Here's the drawing with two shaded views (mm, measured from the low corner). I have some questions. Round coordinates to 2 decimals unless told otherwise and drop trailing zeros. Order: outer loops, then holes, each group sorted by start corner. A loop starts at its lowest first (then second) coordinate and runs counter-clockwise, first axis right, second up. Notation, with made-up numbers: (62.5, -25) -> (114.5, -25) arc R20 ccw to (114.5, -15) -> close; hole circle Ø1 at (16.25, 45.25). An arc over 180 degrees is marked (long way). Answer in a Markdown table with one row per item.
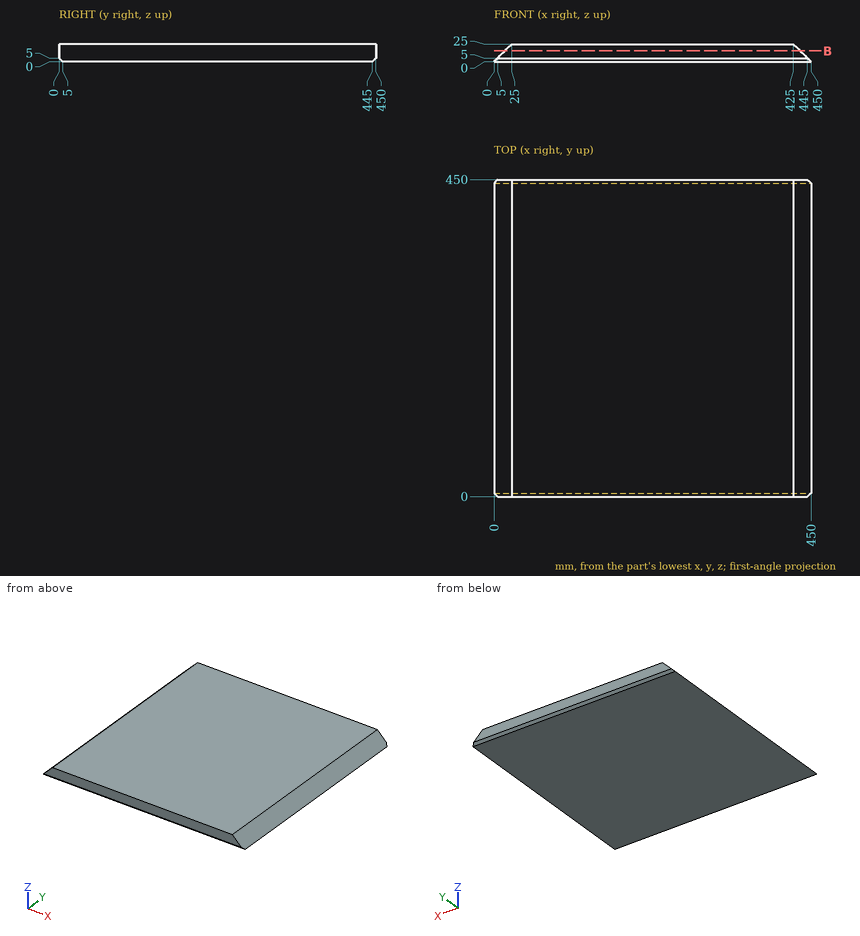
1. For pin 1 Ø10 at (y, z) = (278.5, 17) entering from -X; pin 2 Ø3 at (y, z) = (55.5, 21) entering from -X; pin 3 Ø3 at (y, z) = (396.5, 20) entering from +X, each with a flat end and sliding along its axis, tell me the tip position at first contact or that it passes through.
Numbers:
| item | result |
|---|---|
| pin 1 | stops at x = 12 |
| pin 2 | stops at x = 19.5 |
| pin 3 | stops at x = 431.5 |
2. Suppose I cut it at B-B on z = 15.25. Write out the boundary of the cut face in (x, y), then the cut area to 3 significant figures.
Numbers:
| item | result |
|---|---|
| outline | (15.25, 0) -> (434.75, 0) -> (434.75, 450) -> (15.25, 450) -> close |
| area | 189,000 mm2 |
3. Please list where these lines run through material, in increasing order: line 1 along X through (y, z) = (302.5, 21.25); line 2 along X through (y, z) = (345, 2.5); line 3 along Y through (x, z) = (386.5, 3).
Numbers:
| item | result |
|---|---|
| line 1 | x = 21.25 to 428.75 |
| line 2 | x = 2.5 to 447.5 |
| line 3 | y = 2 to 448 |
